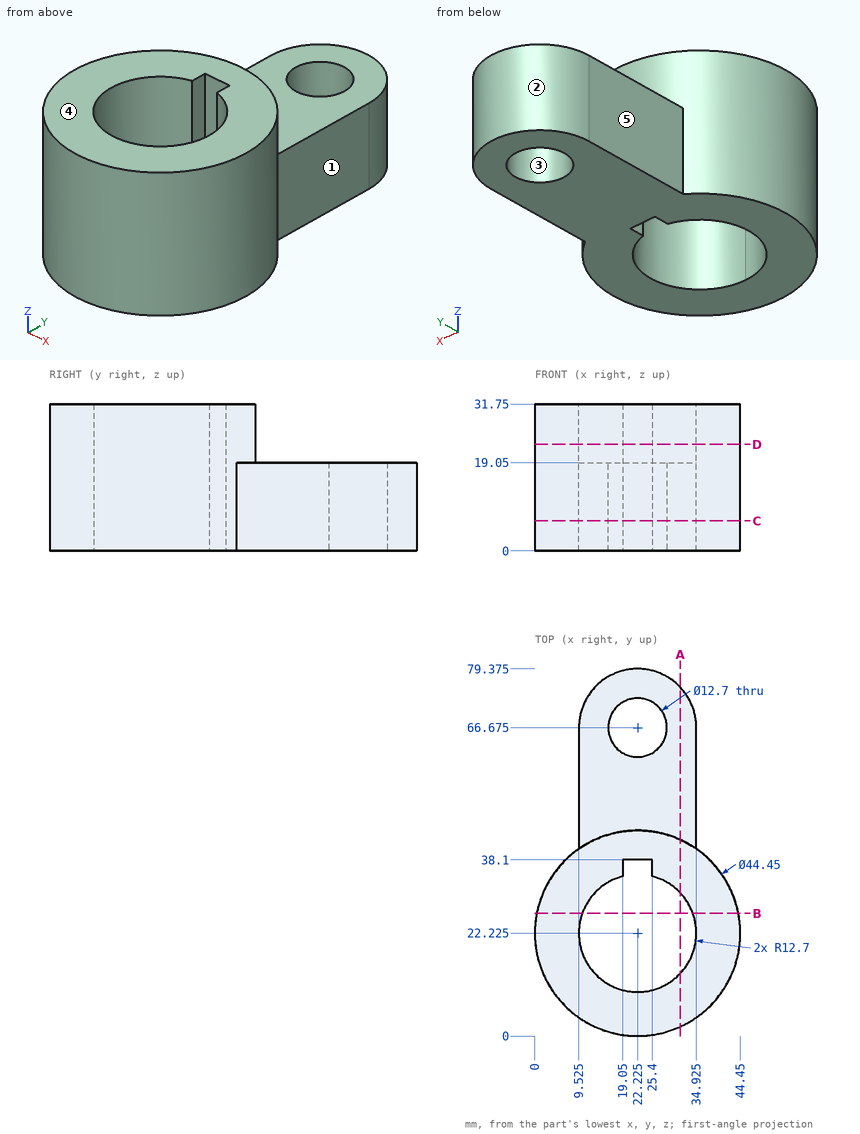
Part print with two shaded views. Sizes in mm from the minimum x, y, z corner. A direction names the side the tool comes from. Round coordinates to 2 decimals unless told otherwise and drop trailing zeros. Order: outer loops, then holes, each group sorted by start corner. A loop starts at its lowest first (then second) coordinate and runs counter-clockwise, first axis right, second up. Notation, with made-up numbers: M 56.25,-10 L 91.25,-10 A23 cw 91.25,26 Z; hole C 10.5,67.25 d3. An arc over 180 degrees is marked long. Answer in a Markdown table with one row per item. Add a question column.
Q1. Cut at C-C on z = 6.5. Give the cut face in (x, y) (3 decimals), and give its area (3 significant figures).
Q2. Mould opens along X. For the marked faces 1, 2 and 3 say: +X half, -X half, draft (parallel to the pull), parting line (faces both ways), or undercut.
Q3. Cut at B-B on y = 26.5. Give the cut face in (x, z), and give its area (3 significant figures).
Q4. 3-axis set-ups, long thin cutter, end or side, ignore diameter. For the marked faces 4 and 5: which of +Z, -Z, +X, -X, +Y, -Y reach the whole face in a straight line?
Q5. Cut at A-A on x = 31.5. Give the cut face in (y, z), and give its area (3 significant figures).
Q6. Wall check: L1, parallel to Y at x = 23.5, z = 17; L2, parallel to X at y = 59, z = 13 (3 decimals); L3, parallel to X at y = 66.5, z = 19 (3 decimals). Give the ranges that are in metal, low to high. Write a range as from..to.
Q7. Cut at D-D on z = 23. Give the cut face in (x, y) (3 decimals), and give its area (3 significant figures).
Q8. Pin check, flat tips, straight feed: pin 1 (1.8 mm diameter, centred on y = 36, z = 20, fed in from +X); pin 2 (9.5 mm diameter, centred on y = 54, z = 8.5, fed in from -X) (3 decimals); pin 3 (12.5 mm diameter, centred on x = 18, y = 63, fed in from +Z); pin 4 (10 mm diameter, centred on x = 22.225, y = 66.675, fed in from -Z). Stop position of each tip, or through.
Established:
| question | item | result |
|---|---|---|
| 1 | outline | M 9.525,40.464 A22.225 ccw long 34.925,40.464 L 34.925,66.675 A12.7 ccw 9.525,66.675 Z; hole C 22.225,66.675 d12.7; hole M 19.05,34.522 A12.7 ccw long 25.4,34.522 L 25.4,38.1 L 19.05,38.1 Z |
| 1 | area | 1,750 mm2 |
| 2 | face 1 | +X half |
| 2 | face 2 | parting line |
| 2 | face 3 | undercut |
| 3 | outline | M 0.42,0 L 10.27,0 L 10.27,31.75 L 0.42,31.75 Z; M 34.18,0 L 44.03,0 L 44.03,31.75 L 34.18,31.75 Z |
| 3 | area | 626 mm2 |
| 4 | face 4 | +Z, +X, -X, +Y, -Y |
| 4 | face 5 | +Z, -Z, -X, +Y |
| 5 | outline | M 2.03,0 L 13.55,0 L 13.55,31.75 L 2.03,31.75 Z; M 30.9,0 L 75.35,0 L 75.35,19.05 L 42.42,19.05 L 42.42,31.75 L 30.9,31.75 Z |
| 5 | area | 1,360 mm2 |
| 6 | L1 | y = 0.04..9.59, 38.1..60.45, 72.9..79.31 |
| 6 | L2 | x = 9.525..34.925 |
| 6 | L3 | x = 9.525..15.877, 28.573..34.925 |
| 7 | outline | C 22.225,22.225 d44.45; hole M 19.05,34.522 A12.7 ccw long 25.4,34.522 L 25.4,38.1 L 19.05,38.1 Z |
| 7 | area | 1,020 mm2 |
| 8 | pin 1 | stops at x = 40.34 |
| 8 | pin 2 | stops at x = 9.525 |
| 8 | pin 3 | stops at z = 19.05 |
| 8 | pin 4 | passes through |
